from build123d import *

# Parameters (mm, degrees)
F0_W     = 1.5
F0_H     = 3
F1_DEPTH = 0.3
F2_DEPTH = 0.6
F3_R     = 4.75
F4_DEPTH = 8
F5_SIZE  = 2.3
F6_SIZE  = 0.29999


# Not quite as in the source:
# - a fillet or chamfer is up to 0.001 mm smaller than in the source, because OpenCascade refuses the exact size


with BuildPart() as f1:
    # F0 (on Front) → F1 (new body)
    with BuildSketch(Plane.XZ):
        with BuildLine():
            Line((8.75, -6), (8.75, 6))
            Line((8.75, 6), (6.3639610307, 6))
            ThreePointArc((6.3639610307, 6), (0, 10.5), (-6.3639610307, 6))
            Line((-6.3639610307, 6), (-8.75, 6))
            Line((-8.75, 6), (-8.75, -6))
            Line((-8.75, -6), (-5, -6))
            Line((-5, -6), (-5, -3))
            Line((-5, -3), (5, -3))
            Line((5, -3), (5, -6))
            Line((5, -6), (8.75, -6))
        make_face()
        with Locations((-6.75, 0)):
            Rectangle(F0_W, F0_H, mode=Mode.SUBTRACT)
        with Locations((6.75, 0)):
            Rectangle(F0_W, F0_H, mode=Mode.SUBTRACT)
        with Locations((-6.75, 0)):
            Rectangle(F0_W, F0_H)
        with Locations((6.75, 0)):
            Rectangle(F0_W, F0_H)
    extrude(amount=F1_DEPTH)

    # F0 (on Front) → F2 (join)
    with BuildSketch(Plane.XZ):
        with Locations((-6.75, 0)):
            Rectangle(F0_W, F0_H)
        with Locations((6.75, 0)):
            Rectangle(F0_W, F0_H)
    extrude(amount=F2_DEPTH)

    # F3 (on face) → F4 (join)
    with BuildSketch(Plane.XZ.offset(0.3)):
        with Locations((0, 3.75)):
            Circle(F3_R)
    extrude(amount=F4_DEPTH)

    # F5
    f5_edges = [f1.edges().sort_by_distance(p)[0] for p in [
        (-4.75, -8.3, 3.75),
    ]]
    chamfer(f5_edges, length=F5_SIZE)

    # F6 (size 0.3 in the source; OpenCascade refuses exactly that, so slightly less here)
    f6_edges = [f1.edges().sort_by_distance(p)[0] for p in [
        (-6.75, -0.6, -1.5),
        (-6.75, -0.6, 1.5),
        (6.75, -0.6, -1.5),
        (6.75, -0.6, 1.5),
        (-5, -0.15, -6),
        (-8.75, -0.15, -6),
        (5, -0.15, -6),
        (8.75, -0.15, -6),
        (8.75, -0.15, 6),
        (-8.75, -0.15, 6),
    ]]
    chamfer(f6_edges, length=F6_SIZE)


solid = f1.part
Input: part model. Units: mm. Frame: model coordinates. A direction names the side the tool comes from. Round coordinates to 2 decimals unless told otherwise and drop trailing zeros. Order: outer loops, then holes, each group sorted by start corner. A loop starts at its lowest first (then second) coordinate and runs counter-clockwise, first axis right, second up. Notation, with made-up numbers: (-13.5, 12) - (6.5, 12) arc R22 cw to (6.5, 23) - close; hole circle Ø3 at (23, 22.25). An arc over 180 degrees is marked (long way). Use a Markdown table: item, result.
1. Section B-B on z = 3.75. Return the cut outline in (x, y).
Evaluation:
| item | result |
|---|---|
| outline | (-8.75, -0.3) - (-4.75, -0.3) - (-4.75, -6) - (-2.45, -8.3) - (2.45, -8.3) - (4.75, -6) - (4.75, -0.3) - (8.75, -0.3) - (8.75, 0) - (-8.75, 0) - close |
2. Access query for faces 1 (the face through (-7, -0.6, 0)), 2 (the face through (2.554, -3.11, 7.755)), 3 (the face through (0, 0, 2)). Directions: +Z, -Z, +X, -X, +Y, -Y. A direction counts if a zero-diameter tool reaches every point of the face in a straight line with its end or side. Return the directions, or none.
Evaluation:
| item | result |
|---|---|
| face 1 | +Z, -Z, -X, -Y |
| face 2 | -Y |
| face 3 | +Z, -Z, +X, -X, +Y |
3. Section D-D on x = 5.75. Return the cut outline in (y, z).
Evaluation:
| item | result |
|---|---|
| outline | (-0.3, -6) - (0, -6) - (0, 7.29) - (-0.3, 7.29) - close |
4. Section C-C on y = -3.5. Return the cut outline in (x, z).
Evaluation:
| item | result |
|---|---|
| outline | circle Ø9.5 at (0, 3.75) |
5. Mould query, pull axis X, two halves, no side actions, for faces 4 (the face through (-0.1, -0.3, -1.3)), 5 (the face through (7, -0.6, 0)), 6 (the face through (0.12, -0.15, 10.5)). Classes: +X half, -X half, draft (parallel to the pull), parting line (faces both ways), or undercut.
Evaluation:
| item | result |
|---|---|
| face 4 | undercut |
| face 5 | draft |
| face 6 | parting line |
6. First-contact query: pin 1 (1.6 mm diameter, centred on x = 7, z = 0, fed in from -Y); pin 2 (3 mm diameter, centred on x = 5, z = 4.5, fed in from -Y); pin 3 (3 mm diameter, centred on x = 4.5, y = -3, fed in from -Z). Flat tips, straight axial feed; report the tip coordinate or a pass-through.
Evaluation:
| item | result |
|---|---|
| pin 1 | y = -0.6 |
| pin 2 | y = -7.19 |
| pin 3 | z = 0.07 |
7. Section A-A on x = 0. Return the cut outline in (y, z), then the cut area to 3 significant figures.
Evaluation:
| item | result |
|---|---|
| outline | (-8.3, 1.3) - (-6, -1) - (-0.3, -1) - (-0.3, -3) - (0, -3) - (0, 10.5) - (-0.3, 10.5) - (-0.3, 8.5) - (-6, 8.5) - (-8.3, 6.2) - close |
| area | 74.8 mm^2 |
8. Material intervals for probe 1 along Y at (x, z) = (4, 6.5); probe 2 along X at (y, z) = (-5.5, 5.25); probe 3 along Z at (x, y) = (2, -1), sorted ascending.
Evaluation:
| item | result |
|---|---|
| probe 1 | -0.3 to 0 |
| probe 2 | -4.51 to 4.51 |
| probe 3 | -0.56 to 8.06 |
